```python
from build123d import *

# Parameters (mm, degrees)
SKETCH1_W           = 10
SKETCH1_H           = 20
BOSS_EXTRUDE1_DEPTH = 16
SKETCH2_W           = 1.4
SKETCH2_H           = 4.3
CUT_EXTRUDE1_DEPTH  = 5
CUT_EXTRUDE2_DEPTH  = 10
FILLET2_R           = 1


with BuildPart() as part:
    # Sketch1 → Boss-Extrude1 (new body)
    with BuildSketch(Plane(origin=(0, 0, 0), x_dir=(1, 0, 0), z_dir=(0, 1, 0))):
        Rectangle(SKETCH1_W, SKETCH1_H)
    extrude(amount=BOSS_EXTRUDE1_DEPTH)

    # Sketch2 → Cut-Extrude1 (cut)
    with BuildSketch(Plane.XZ):
        Rectangle(SKETCH2_W, SKETCH2_H)
    extrude(amount=-CUT_EXTRUDE1_DEPTH, mode=Mode.SUBTRACT)

    # Sketch6 → Cut-Extrude2 (cut)
    with BuildSketch(Plane(origin=(5, 0, 0), x_dir=(0, 0, -1), z_dir=(1, 0, 0))):
        with BuildLine():
            Line((-6, 16), (6, 16))
            ThreePointArc((6, 16), (0, 14.36598161), (-6, 16))
        make_face()
    extrude(amount=-CUT_EXTRUDE2_DEPTH, mode=Mode.SUBTRACT)

    # Fillet2
    fillet2_edges = [part.edges().sort_by_distance(p)[0] for p in [
        (0, 16, 10),
        (5, 8, 10),
        (-5, 8, 10),
        (-5, 8, -10),
        (5, 8, -10),
        (0, 16, -10),
    ]]
    fillet(fillet2_edges, radius=FILLET2_R)


solid = part.part
```
Work out the finished part from the listing and answer in its coordinate system (mm). A direction names the side the tool comes from. Coordinates: 2 decimals unless noted, no trailing zeros. Order: outer loops, then holes, each group sorted by start corner. A loop starts at its lowest first (then second) coordinate and runs counter-clockwise, first axis right, second up. Notation, with made-up numbers: (85, -26) - (123, -26) arc R19 ccw to (123, -12) - close; hole circle Ø7 at (7, 46.25). An arc over 180 degrees is marked (long way). Answer as a JSON object with one key per item and string values.
1. Find section A-A on x = -1.5. Determine the outline of the cut face in (y, z), plus the area to 3 significant figures.
Output values:
{"outline": "(0, -10) - (15, -10) arc R1 ccw to (16, -9) - (16, -6) arc R11.83 cw to (16, 6) - (16, 9) arc R1 ccw to (15, 10) - (0, 10) - close", "area": "306 mm²"}
2. The mould has two halves that part along X. Classify faces 3 (the face through (4.699, 8.112, 9.715)), 4 (the face through (0.07, 15.715, 9.699)), 5 (the face through (0, 2, -2.15)), 6 (the face through (0, 5, 0)): +X half, -X half, draft (parallel to the pull), parting line (faces both ways), or undercut.
Output values:
{"face 3": "+X half", "face 4": "draft", "face 5": "undercut", "face 6": "undercut"}
3. Find section C-C on z = -0.5. Determine the outline of the cut face in (x, y), plus the area to 3 significant figures.
Output values:
{"outline": "(-5, 0) - (-0.7, 0) - (-0.7, 5) - (0.7, 5) - (0.7, 0) - (5, 0) - (5, 14.38) - (-5, 14.38) - close", "area": "137 mm²"}
4. A tool of negligible diameter and unlimited length cuts with its end or side. For faces 1 (the face through (0.7, 2, 0)), 2 (the face through (0.07, 14.366, -0.088)), from which of +Z, -Z, +X, -X, +Y, -Y can it reach the whole face along a straight path? Write none if from no direction.
Output values:
{"face 1": "-Y", "face 2": "+X, -X, +Y"}
5. Find section D-D on z = 2.5. Determine the outline of the cut face in (x, y).
Output values:
{"outline": "(-5, 0) - (5, 0) - (5, 14.63) - (-5, 14.63) - close"}
6. Find section B-B on y = 4.5. Determine the outline of the cut face in (x, z).
Output values:
{"outline": "(-5, -9) arc R1 ccw to (-4, -10) - (4, -10) arc R1 ccw to (5, -9) - (5, 9) arc R1 ccw to (4, 10) - (-4, 10) arc R1 ccw to (-5, 9) - close; hole (-0.7, -2.15) - (0.7, -2.15) - (0.7, 2.15) - (-0.7, 2.15) - close"}
7. Consider line 1 (Z direction, x = 0.5, y = 1.25); line 2 (Z direction, x = -2, y = 15.25); line 3 (Y direction, x = 0, z = 4.25). Determine where each line is inside the solid, lowest interval first.
Output values:
{"line 1": "z = -10 to -2.15, 2.15 to 10", "line 2": "z = -9.97 to -4.49, 4.49 to 9.97", "line 3": "y = 0 to 15.16"}
